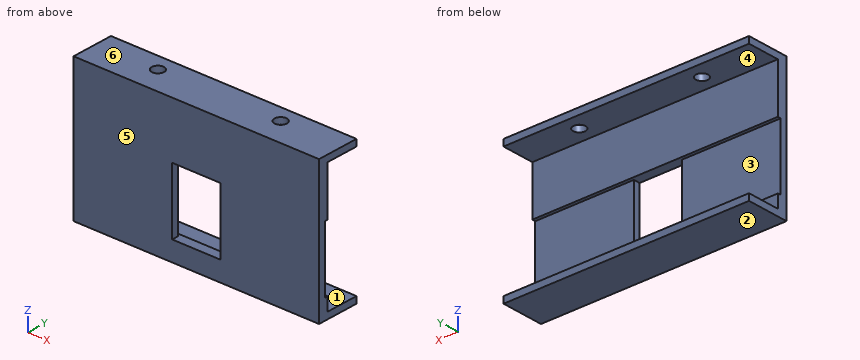
from build123d import *

# Parameters (mm, degrees)
SKETCH1_W           = 75
SKETCH1_H           = 43
BOSS_EXTRUDE1_DEPTH = 3
SKETCH2_W           = 75
SKETCH2_H           = 2
BOSS_EXTRUDE2_DEPTH = 10
SKETCH3_W           = 75
SKETCH3_H           = 2
BOSS_EXTRUDE3_DEPTH = 10
SKETCH4_OUTSIDE_W   = 94.484
SKETCH4_OUTSIDE_H   = 32.484
SKETCH4_OUTSIDE_W_2 = 79
SKETCH4_OUTSIDE_H_2 = 17
SKETCH4_OUTSIDE_R   = 1.875
CUT_EXTRUDE2_DEPTH  = 2
SKETCH6_W           = 14.75
SKETCH6_H           = 20
CUT_EXTRUDE3_DEPTH  = 45.367781103
SKETCH7_W           = 75
SKETCH7_H           = 20
CUT_EXTRUDE4_DEPTH  = 1


with BuildPart() as part:
    # Sketch1 → Boss-Extrude1 (new body)
    with BuildSketch(Plane(origin=(0, 0, 0), x_dir=(1, 0, 0), z_dir=(0, 1, 0))):
        Rectangle(SKETCH1_W, SKETCH1_H)
    extrude(amount=BOSS_EXTRUDE1_DEPTH)

    # Sketch2 → Boss-Extrude2 (add)
    with BuildSketch(Plane(origin=(0, 3, 0), x_dir=(1, 0, 0), z_dir=(0, 1, 0))):
        with Locations((0, 20.5)):
            Rectangle(SKETCH2_W, SKETCH2_H)
    extrude(amount=BOSS_EXTRUDE2_DEPTH)

    # Sketch3 → Boss-Extrude3 (add)
    with BuildSketch(Plane(origin=(0, 3, 0), x_dir=(1, 0, 0), z_dir=(0, 1, 0))):
        with Locations((0, -20.5)):
            Rectangle(SKETCH3_W, SKETCH3_H)
    extrude(amount=BOSS_EXTRUDE3_DEPTH)

    # Sketch4 outside → Cut-Extrude2 (cut)
    # profile 1 of 3: a face of its own
    with BuildSketch(Plane.XY.offset(21.5)):
        with Locations((0, 6.5)):
            Rectangle(SKETCH4_OUTSIDE_W, SKETCH4_OUTSIDE_H)
        with Locations((0, 6.5)):
            Rectangle(SKETCH4_OUTSIDE_W_2, SKETCH4_OUTSIDE_H_2, mode=Mode.SUBTRACT)
    # profile 2 of 3: a face of its own
    with BuildSketch(Plane.XY.offset(21.5)):
        with Locations((18.75, 8)):
            Circle(SKETCH4_OUTSIDE_R)
    # profile 3 of 3: a face of its own
    with BuildSketch(Plane.XY.offset(21.5)):
        with Locations((-18.75, 8)):
            Circle(SKETCH4_OUTSIDE_R)
    extrude(amount=-CUT_EXTRUDE2_DEPTH, mode=Mode.SUBTRACT)

    # Sketch6 → Cut-Extrude3 (cut, through all)
    with BuildSketch(Plane(origin=(0, 3, 0), x_dir=(1, 0, 0), z_dir=(0, 1, 0))):
        with Locations((0, 5.5)):
            Rectangle(SKETCH6_W, SKETCH6_H)
    extrude(amount=-CUT_EXTRUDE3_DEPTH, mode=Mode.SUBTRACT)

    # Sketch7 → Cut-Extrude4 (cut)
    with BuildSketch(Plane(origin=(0, 3, 0), x_dir=(1, 0, 0), z_dir=(0, 1, 0))):
        with Locations((0, 5.5)):
            Rectangle(SKETCH7_W, SKETCH7_H)
    extrude(amount=-CUT_EXTRUDE4_DEPTH, mode=Mode.SUBTRACT)


solid = part.part
Could you check a few things on this model? Use its own coordinates, in mm. Face numbers are marked on the shaded views. A direction names the side the tool comes from. Coordinates: 2 decimals unless noted, no trailing zeros. Write each loop counter-clockwise with the first axis right and the second up, starting at its lowest first coordinate (ties: lowest second). Pieces come first, ordered by that corner, then holes. Notation, with made-up numbers: M 44.5,-38.75 L 50.5,-38.75 A4 cw 50.5,-32.75 Z; hole C 50,84.25 d3. An arc over 180 degrees is marked long. One line per question, with ' | ' between items.
1) Imagine slicing it at A-A, the plane z = -9.5. Write out the boundary of the cut face in (x, y) (3 decimals).
Checks:
outline: M -37.5,0 L -7.375,0 L -7.375,2 L -37.5,2 Z; M 7.375,0 L 37.5,0 L 37.5,2 L 7.375,2 Z
2) If we mould it in two halves opening along Z, with no side actions, what happens to the marked faces 3, 4, 5 and 6? For each: released by +Z, released by -Z, zero draft, split by the parting line, or undercut.
Checks:
face 3: undercut | face 4: undercut | face 5: zero draft | face 6: released by +Z
3) I need wall thicknesses on probe 1 along Z at (x, y) = (34.5, 11.5); probe 2 along Y at (x, z) = (-18.75, 21.05) (3 decimals); probe 3 along Z at (x, y) = (-28.5, 2.75). Which ranges of each line are inside material? Lowest first, please. Write a range as [from, to].
Checks:
probe 1: [-21.5, -19.5], [19.5, 21.5] | probe 2: [0, 6.125], [9.875, 13] | probe 3: [-21.5, -15.5], [4.5, 21.5]
4) For the marked faces 1 and 2, which set-ups out of +Z, -Z, +X, -X, +Y, -Y let a thin tool reach every point of the face, with its end or its side?
Checks:
face 1: +X, -X, +Y | face 2: -Z, +X, -X, +Y, -Y
5) Imagine slicing it at D-D, the plane x = -27.5. Write out the boundary of the cut face in (y, z), and give its area (3 significant figures).
Checks:
outline: M 0,-21.5 L 13,-21.5 L 13,-19.5 L 3,-19.5 L 3,-15.5 L 2,-15.5 L 2,4.5 L 3,4.5 L 3,19.5 L 13,19.5 L 13,21.5 L 0,21.5 Z | area: 149 mm²
6) Imagine slicing it at B-B, the plane x = -18.75. Write out the boundary of the cut face in (y, z) (3 decimals), and give its area (4 significant figures).
Checks:
outline: M 0,-21.5 L 13,-21.5 L 13,-19.5 L 3,-19.5 L 3,-15.5 L 2,-15.5 L 2,4.5 L 3,4.5 L 3,19.5 L 6.125,19.5 L 6.125,21.5 L 0,21.5 Z; M 9.875,19.5 L 13,19.5 L 13,21.5 L 9.875,21.5 Z | area: 141.5 mm²
7) For pin 1 Ø6 at (x, z) = (20.5, -2.5) entering from +Y; pin 2 Ø12 at (x, z) = (24, -12) entering from +Y; pin 3 Ø2 at (x, y) = (-18.75, 8) entering from +Z, each with a flat end and sliding along its axis, tell me the tip position at first contact or that it passes through.
Checks:
pin 1: y = 2 | pin 2: y = 3 | pin 3: z = -19.5
8) Imagine slicing it at C-C, the plane y = 5.25. Write out the boundary of the cut face in (x, z).
Checks:
outline: M -37.5,-21.5 L 37.5,-21.5 L 37.5,-19.5 L -37.5,-19.5 Z; M -37.5,19.5 L 37.5,19.5 L 37.5,21.5 L -37.5,21.5 Z
